```python
from build123d import *

# Parameters (mm, degrees)
F0_R     = 12.7
F1_DEPTH = 50.8
F3_DEPTH = 76.2
F4_R     = 38.1
F5_DEPTH = 12.7
F6_R     = 9.525
F7_DEPTH = 42.418


# Not quite as in the source:
# - the program builds the solid bodies; features that only make, move or delete a surface that nothing else refers to are left out


with BuildPart() as f1:
    # F0 (on Front) → F1 (new body, symmetric)
    with BuildSketch(Plane.XZ):
        with BuildLine():
            Line((154.00903388, 91.1349219612), (-142.45976612, 91.1349219612))
            ThreePointArc((-142.45976612, 91.1349219612), (-201.7060726901, 107.0099219612), (-158.33476612, 63.638615391))
            Line((-158.33476612, 63.638615391), (-86.30036612, -61.1286253017))
            ThreePointArc((-86.30036612, -61.1286253017), (-86.30036612, -116.121238442), (-38.67536612, -88.6249318719))
            Line((-38.67536612, -88.6249318719), (50.22463388, -88.6249318719))
            ThreePointArc((50.22463388, -88.6249318719), (97.84963388, -116.121238442), (97.84963388, -61.1286253017))
            Line((97.84963388, -61.1286253017), (169.88403388, 63.638615391))
            ThreePointArc((169.88403388, 63.638615391), (213.2553404502, 107.0099219612), (154.00903388, 91.1349219612))
        make_face()
        with Locations((-70.42536612, -88.6249318719)):
            Circle(F0_R, mode=Mode.SUBTRACT)
        with Locations((81.97463388, -88.6249318719)):
            Circle(F0_R, mode=Mode.SUBTRACT)
        with Locations((-174.20976612, 91.1349219612)):
            Circle(F0_R, mode=Mode.SUBTRACT)
        with Locations((185.75903388, 91.1349219612)):
            Circle(F0_R, mode=Mode.SUBTRACT)
    extrude(amount=-F1_DEPTH, both=True)

    # F2 (on face) → F3 (cut)
    with BuildSketch(Plane(origin=(0, 50.8, 0), x_dir=(-1, 0, 0), z_dir=(0, 1, 0))):
        Polygon((122.883327189, 91.1349219612), (-134.4325949491, 91.1349219612), (-58.2325949491, -40.8473495756), (46.683327189, -40.8473495756), align=None)
    extrude(amount=-F3_DEPTH, mode=Mode.SUBTRACT)

    # F4 (on Front) → F5 (cut, symmetric)
    with BuildSketch(Plane.XZ):
        with Locations((186.0332787037, 91.5846452117)):
            Circle(F4_R)
    extrude(amount=F5_DEPTH, both=True, mode=Mode.SUBTRACT)

    # F6 (on face) → F7 (cut, symmetric)
    with BuildSketch(Plane(origin=(0, -25.4, 0), x_dir=(-1, 0, 0), z_dir=(0, 1, 0))):
        with BuildLine():
            ThreePointArc((47.625, 0), (38.1, 9.525), (28.575, 0))
            ThreePointArc((28.575, 0), (38.1, -9.525), (47.625, 0))
        make_face()
        with Locations((-38.1, 0)):
            Circle(F6_R)
    extrude(amount=F7_DEPTH, both=True, mode=Mode.SUBTRACT)


solid = f1.part
```
Geometry check sheet. Reference: the model listing, model coordinates, mm. A direction names the side the tool comes from. Round coordinates to 2 decimals unless told otherwise and drop trailing zeros. Order: outer loops, then holes, each group sorted by start corner. A loop starts at its lowest first (then second) coordinate and runs counter-clockwise, first axis right, second up. Notation, with made-up numbers: (-33.5, -37) - (-20.5, -37) arc R19 cw to (-20.5, -4) - close; hole circle Ø7 at (84.25, 29). An arc over 180 degrees is marked (long way). Use a Markdown table: item, result. Add a question column.
1) Mould release check, pull along Y, two halves, no side actions. Record for faces 1 (the flat face through (175, 12.7, 84)), 2 (the cylindrical face through (-29.015, -37.922, -2.861)), 3 (the cylindrical face through (153, -0.2, 72.6)), 4 (the flat face through (-11, 50.8, -43)): released by +Y, released by -Y, zero draft, split by the parting line, or undercut.
2) Section check B-B (y = 20). Record the cut outline in (x, z).
3) Gauge pin test, flat ends, axial feed: P1, Ø2, axis at y = 40.5, z = -22.5, coming from the -X side; P2, Ø23, axis at x = -13, y = 23, coming from the +Z side; P3, Ø2, axis at y = -15, z = 78.5, coming from the +X side. Record the tip position at first contact, or that the pin passes through.
4) Thickness scan on line 1 along Y through (x, z) = (162, 96); line 2 along Z through (x, y) = (-38.1, -42.5) (3 decimals); line 3 along X through (y, z) = (10, 89). Record the ranges inside material, lowest first.
5) Section check D-D (y = 1). Record the cut outline in (x, z), then the cut area to 3 significant figures.
6) Section check C-C (z = -81). Record the cut outline in (x, y), then the cut area to 3 significant figures.
7) Set-up check for faces 5 (the flat face through (5, 1, -88.625)), 6 (the flat face through (8, -33, 91.135)), 7 (the flat face through (-84.25, 13.23, 24.22)): record each of +Z, -Z, +X, -X, +Y, -Y from which the full face is reachable in a straight line by a thin tool's end or side.
8) Section check A-A (x = 38.1). Record the cut outline in (y, z) (3 decimals).
Established:
| question | item | result |
|---|---|---|
| 1 | face 1 | undercut |
| 1 | face 2 | zero draft |
| 1 | face 3 | undercut |
| 1 | face 4 | released by +Y |
| 2 | outline | (-158.33, 63.64) - (-86.3, -61.13) arc R31.75 ccw (long way) to (-38.68, -88.62) - (50.22, -88.62) arc R31.75 ccw (long way) to (97.85, -61.13) - (169.88, 63.64) arc R31.75 ccw (long way) to (154.01, 91.13) - (134.43, 91.13) - (58.23, -40.85) - (-46.68, -40.85) - (-122.88, 91.13) - (-142.46, 91.13) arc R31.75 ccw (long way) to start; hole circle Ø25.4 at (-174.21, 91.13); hole circle Ø25.4 at (-70.43, -88.62); hole circle Ø25.4 at (81.97, -88.62); hole circle Ø25.4 at (185.76, 91.13) |
| 3 | P1 | x = -109.18 |
| 3 | P2 | z = -40.85 |
| 3 | P3 | x = 215.3 |
| 4 | line 1 | -50.8 to -12.7, 12.7 to 50.8 |
| 4 | line 2 | -88.625 to -9.525, 9.525 to 91.135 |
| 4 | line 3 | -205.89 to -186.73, -161.69 to -121.65, 133.2 to 148.02 |
| 5 | outline | (-158.33, 63.64) - (-86.3, -61.13) arc R31.75 ccw (long way) to (-38.68, -88.62) - (50.22, -88.62) arc R31.75 ccw (long way) to (97.85, -61.13) - (166.97, 58.6) arc R38.1 cw to (147.94, 91.13) - (134.43, 91.13) - (58.23, -40.85) - (-46.68, -40.85) - (-122.88, 91.13) - (-142.46, 91.13) arc R31.75 ccw (long way) to start; hole circle Ø25.4 at (-174.21, 91.13); hole circle Ø25.4 at (-70.43, -88.62); hole circle Ø25.4 at (81.97, -88.62) |
| 5 | area | 26,700 mm2 |
| 6 | outline | (-101.25, -50.8) - (-80.58, -50.8) - (-80.58, 50.8) - (-101.25, 50.8) - close; (-60.27, -50.8) - (71.82, -50.8) - (71.82, 50.8) - (-60.27, 50.8) - close; (92.13, -50.8) - (112.8, -50.8) - (112.8, 50.8) - (92.13, 50.8) - close |
| 6 | area | 17,600 mm2 |
| 7 | face 5 | -Z, +Y, -Y |
| 7 | face 6 | +Z, +Y, -Y |
| 7 | face 7 | +Z, +Y |
| 8 | outline | (-50.8, -88.625) - (50.8, -88.625) - (50.8, -40.847) - (-25.4, -40.847) - (-25.4, -9.525) - (-50.8, -9.525) - close; (-50.8, 9.525) - (-25.4, 9.525) - (-25.4, 91.135) - (-50.8, 91.135) - close |
